Source: CAD feature listing. Evaluate the final solid. Frame: model axes, mm. Coordinates: 2 decimals unless noted, no trailing zeros. Loops run counter-clockwise (first coordinate to the right, second up) from the corner with the lowest first, then second, coordinate; pieces in that order, holes last. Notation, with made-up numbers: (-1, -15) - (16, -15) arc R3 cw to (16, -10) - close; hole circle Ø7 at (74.5, 65). An arc over 180 degrees is marked (long way). Write item = value, one per line. Start each with the question number.
from build123d import *

# Parameters (mm, degrees)
BOSS_EXTRUDE1_DEPTH = 2.3622
SKETCH2_R           = 2
SKETCH2_R_2         = 3.75
SKETCH2_R_3         = 1.5
SKETCH2_R_4         = 15.5
CUT_EXTRUDE1_DEPTH  = 292.557164187


with BuildPart() as part:
    # Sketch1 → Boss-Extrude1 (new body)
    with BuildSketch(Plane.XY):
        Polygon((0, 0), (150, 0), (150, 20), (147.6378, 20), (147.6378, 40), (150, 40), (150, 74.740014023), (147.6378, 74.740014023), (147.6378, 94.740014023), (150, 94.740014023), (150, 114.740014023), (135.227883705, 117.344736688), (134.81769198, 115.018423813), (124.969614449, 116.75490559), (125.379806175, 119.081218464), (100.759612349, 123.422422906), (100.349420624, 121.096110032), (90.501343094, 122.832591808), (90.911534819, 125.158904683), (76.139418524, 127.763627348), (71.95711156, 147.321446972), (69.647137484, 146.827474696), (65.464830521, 166.385294321), (67.774804596, 166.879266596), (58.364613928, 210.884360751), (56.054639852, 210.390388476), (51.872332888, 229.9482081), (54.182306964, 230.442180376), (50, 250), (35, 250), (35, 247.6378), (15, 247.6378), (15, 250), (0, 250), (0, 230), (2.3622, 230), (2.3622, 210), (0, 210), (0, 135), (2.3622, 135), (2.3622, 115), (0, 115), (0, 40), (2.3622, 40), (2.3622, 20), (0, 20), align=None)
    extrude(amount=BOSS_EXTRUDE1_DEPTH)

    # Sketch2 → Cut-Extrude1 (cut, through all)
    with BuildSketch(Plane.XY.offset(2.3622)):
        with Locations((30, 168.301817255)):
            Circle(SKETCH2_R)
        with Locations((67.180515984, 70)):
            Circle(SKETCH2_R)
        with Locations((46, 43.014719635)):
            Circle(SKETCH2_R)
        with Locations((67.180515984, 105)):
            Circle(SKETCH2_R)
        with Locations((25, 43.014719635)):
            Circle(SKETCH2_R)
        with Locations((30, 205.319678906)):
            Circle(SKETCH2_R)
        with Locations((30, 134.64241622)):
            Circle(SKETCH2_R)
        with Locations((110, 13.75)):
            Circle(SKETCH2_R_2)
        with Locations((89.4, 22.5)):
            Circle(SKETCH2_R_3)
        with Locations((89.4, 5)):
            Circle(SKETCH2_R_3)
        with Locations((107.457467604, 56.31719907)):
            Circle(SKETCH2_R_4)
        with BuildLine():
            Line((41, 105), (41, 70))
            ThreePointArc((41, 70), (39, 68), (37, 70))
            Line((37, 70), (37, 105))
            ThreePointArc((37, 105), (39, 107), (41, 105))
        make_face()
        with BuildLine():
            Line((48, 105), (48, 70))
            ThreePointArc((48, 70), (46, 68), (44, 70))
            Line((44, 70), (44, 105))
            ThreePointArc((44, 105), (46, 107), (48, 105))
        make_face()
        with BuildLine():
            Line((34, 105), (34, 70))
            ThreePointArc((34, 70), (32, 68), (30, 70))
            Line((30, 70), (30, 105))
            ThreePointArc((30, 105), (32, 107), (34, 105))
        make_face()
        with BuildLine():
            Line((27, 105), (27, 70))
            ThreePointArc((27, 70), (25, 68), (23, 70))
            Line((23, 70), (23, 105))
            ThreePointArc((23, 105), (25, 107), (27, 105))
        make_face()
    extrude(amount=-CUT_EXTRUDE1_DEPTH, mode=Mode.SUBTRACT)


solid = part.part
Item 1: Cut plane D-D (y = 142). Return the cut outline in (x, z).
Item 2: Material intervals for L1, parallel to X at y = 74.5, z = 0.1; L2, parallel to Y at x = 89.4, z = 1.55; L3, parallel to X at y = 57, z = 2.05, sorted ascending. Write a range as [from, to].
Item 3: Cut plane C-C (y = 200.5). Return the cut outline in (x, z), then the cut area to 3 significant figures.
Item 4: Cut plane B-B (z = 0.6). State how many separate pieces and enclosed holes the cut face has, then the cut area to 3 significant figures.
Item 5: First-contact query: pin 1 (1.5 mm diameter, centred on x = 67.5, y = 44, fed in from -Z); pin 2 (0.7 mm diameter, centred on x = 28, z = 1, fed in from +Y); pin 3 (1.2 mm diameter, centred on y = 92.5, z = 2, fed in from +X). Flat tips, straight axial feed; report the tip coordinate or a pass-through.
Item 6: Cut plane A-A (y = 13.75). Return the cut outline in (x, z), then the cut area to 3 significant figures.
Item 7: Draft query along X for faces 1 (the cylindrical face through (107, 11.5, 1.2)), 2 (the flat face through (57, 99, 2.362)), 3 (the flat face through (63.136, 188.574, 1.165)). Return one class per face: released by +X, released by -X, zero draft, split by the parting line, or undercut.
Responses:
q1.outline = (0, 0) - (73.1, 0) - (73.1, 2.36) - (0, 2.36) - close
q2.L1 = [0, 23], [27, 30], [34, 37], [41, 44], [48, 150]
q2.L2 = [0, 3.5], [6.5, 21], [24, 125.43]
q2.L3 = [0, 91.97], [122.94, 150]
q3.outline = (0, 0) - (60.59, 0) - (60.59, 2.36) - (0, 2.36) - close
q3.area = 143 mm2
q4.separate_pieces = 1
q4.enclosed_holes = 15
q4.area = 24,500 mm2
q5.pin_1 = 0
q5.pin_2 = 247.64
q5.pin_3 = 147.64
q6.outline = (0, 0) - (106.25, 0) - (106.25, 2.36) - (0, 2.36) - close; (113.75, 0) - (150, 0) - (150, 2.36) - (113.75, 2.36) - close
q6.area = 337 mm2
q7.face_1 = undercut
q7.face_2 = zero draft
q7.face_3 = released by +X
